from build123d import *

# Parameters (mm, degrees)
CROQUIS1_R                   = 3
SALIENTE_EXTRUIR1_DEPTH      = 18
CROQUIS1_2_R                 = 3
SALIENTE_EXTRUIR2_DEPTH      = 21.5
SALIENTE_EXTRUIR2_DEPTH_BACK = 1.5
CROQUIS3_R                   = 3
CORTAR_EXTRUIR1_DEPTH        = 4
CROQUIS9_R                   = 1.125
SALIENTE_EXTRUIR3_DEPTH      = 55
CROQUIS10_R                  = 0.75
SALIENTE_EXTRUIR4_DEPTH      = 110


with BuildPart() as part:
    # Croquis1 → Saliente-Extruir1 (new body)
    with BuildSketch(Plane.XY):
        Circle(CROQUIS1_R)
    extrude(amount=SALIENTE_EXTRUIR1_DEPTH)

    # Croquis1_2 → Saliente-Extruir2 (add, two sides)
    with BuildSketch(Plane.XY) as saliente_extruir2_sk:
        Circle(CROQUIS1_2_R)
    extrude(amount=SALIENTE_EXTRUIR2_DEPTH)
    extrude(saliente_extruir2_sk.sketch, amount=-SALIENTE_EXTRUIR2_DEPTH_BACK)

    # Croquis3 → Cortar-Extruir1 (cut)
    with BuildSketch(Plane(origin=(0, 0, -1.5), x_dir=(-1, 0, 0), z_dir=(0, 0, -1))):
        Circle(CROQUIS3_R)
    extrude(amount=-CORTAR_EXTRUIR1_DEPTH, mode=Mode.SUBTRACT)

    # Croquis9 → Saliente-Extruir3 (add)
    with BuildSketch(Plane.XY.offset(21.5)):
        with Locations((0, -1.15)):
            Circle(CROQUIS9_R)
        with Locations((0, 1.15)):
            Circle(CROQUIS9_R)
    extrude(amount=SALIENTE_EXTRUIR3_DEPTH)

    # Croquis10 → Saliente-Extruir4 (add)
    with BuildSketch(Plane.XY.offset(21.5)):
        with Locations((0, -1.15)):
            Circle(CROQUIS10_R)
        with Locations((0, 1.15)):
            Circle(CROQUIS10_R)
    extrude(amount=SALIENTE_EXTRUIR4_DEPTH)


solid = part.part
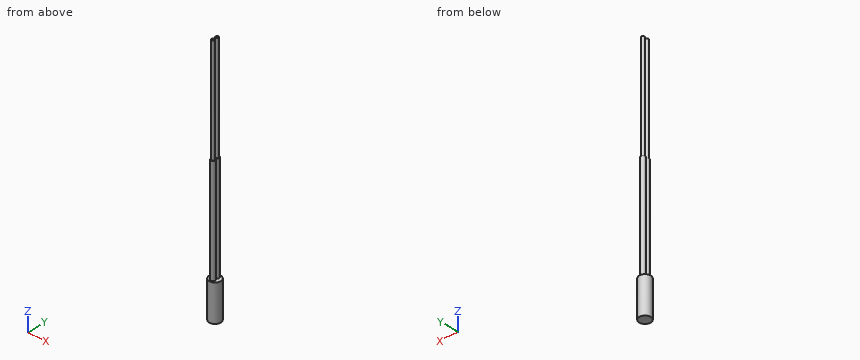
Could you check a few things on this model? Use its own coordinates, in mm. Give positions to 0.01 mm unless a question says otherwise; leave off trailing zeros. Loops run counter-clockwise (first coordinate to the right, second up) from the corner with the lowest first, then second, coordinate; pieces in that order, holes last. Notation, with made-up numbers: M 59,-19 L 74,-19 A15 cw 74,-5 Z; hole C 83,-5 d8. An arc over 180 degrees is marked long. Answer as a JSON object with one key per item and string values.
Q1. If I drill on probe 1 along Z at (x, y) = (0.3, -2.4); probe 2 along X at (y, z) = (-2, 35.5); probe 3 along Y at (x, z) = (-2.3, 12), over which ranges is the centre line in solid material (lowest first)? Write a range as [from, to].
Values found:
{"probe 1": "z = [2.5, 21.5]", "probe 2": "x = [-0.74, 0.74]", "probe 3": "y = [-1.93, 1.93]"}
Q2. For P1, Ø1, axis at x = 0.5, z = 70.5, coming from the +Y side (3 decimals); P2, Ø3, axis at y = -2, z = 58, coming from the -X side (3 decimals); P3, Ø3, axis at x = -0.5, z = 39.5, coming from the -Y side (3 decimals); P4, Ø3, axis at x = -1, y = 0.5, coming from the +Z side, each with a flat end and sliding along its axis, tell me the tip position at first contact or that it passes through.
Values found:
{"P1": "stops at y = 2.275", "P2": "stops at x = -1.125", "P3": "stops at y = -2.275", "P4": "stops at z = 131.5"}
Q3. Suppose I cut it at A-A, the plane z = 95.5. List the corners of the cut face in (x, y) for me, plus the area to 3 significant figures.
Values found:
{"outline": "C 0,-1.15 d1.5; C 0,1.15 d1.5", "area": "3.53 mm²"}
Q4. Suppose I cut it at B-B, the plane z = 17. List the corners of the cut face in (x, y) for me.
Values found:
{"outline": "C 0,0 d6"}
